For this review, take the finished solid that the model builds, in its own axes (mm). A direction names the side the tool comes from. Coordinates: 2 decimals unless noted, no trailing zeros. Write each loop counter-clockwise with the first axis right and the second up, starting at its lowest first coordinate (ties: lowest second). Pieces come first, ordered by that corner, then holes. Notation, with made-up numbers: (-22, 41.25) - (28, 41.25) arc R17 ccw to (28, 56.25) - close; hole circle Ø10 at (46, -25.5). An arc over 180 degrees is marked (long way). Write each question's results on one line, items separated by ' | '.
from build123d import *

# Parameters (mm, degrees)
SKETCH_1_W          = 41
SKETCH_1_H          = 19
EXTRUDE_2_DEPTH     = 2
SKETCH_2_W          = 41
SKETCH_2_H          = 2
EXTRUDE_3_DEPTH     = 25
SKETCH_3_R          = 2
CUT_EXTRUDE_1_DEPTH = 25
FILLET_1_R          = 1
FILLET_2_R          = 1
FILLET_3_R          = 1
FILLET_4_R          = 1
FILLET_5_R          = 1
FILLET_6_R          = 1


with BuildPart() as part:
    # 草图1 → 凸台-拉伸2 (new body)
    with BuildSketch(Plane(origin=(0, 0, 0), x_dir=(1, 0, 0), z_dir=(0, 1, 0))):
        Rectangle(SKETCH_1_W, SKETCH_1_H)
    extrude(amount=EXTRUDE_2_DEPTH)

    # 草图2 → 凸台-拉伸3 (add)
    with BuildSketch(Plane(origin=(0, 2, 0), x_dir=(1, 0, 0), z_dir=(0, 1, 0))):
        with Locations((0, 8.5)):
            Rectangle(SKETCH_2_W, SKETCH_2_H)
    extrude(amount=EXTRUDE_3_DEPTH)

    # 草图3 → 切除-拉伸1 (cut)
    with BuildSketch(Plane.XY.offset(-7.5)):
        with Locations((-12.5, 19)):
            Circle(SKETCH_3_R)
        with Locations((12.5, 19)):
            Circle(SKETCH_3_R)
    extrude(amount=-CUT_EXTRUDE_1_DEPTH, mode=Mode.SUBTRACT)

    # 圆角1
    fillet_1_edges = [part.edges().sort_by_distance(p)[0] for p in [
        (0, 2, -7.5),
    ]]
    fillet(fillet_1_edges, radius=FILLET_1_R)

    # 圆角2
    fillet_2_edges = [part.edges().sort_by_distance(p)[0] for p in [
        (0, 0, -9.5),
    ]]
    fillet(fillet_2_edges, radius=FILLET_2_R)

    # 圆角3
    fillet_3_edges = [part.edges().sort_by_distance(p)[0] for p in [
        (-20.5, 1, 9.5),
    ]]
    fillet(fillet_3_edges, radius=FILLET_3_R)

    # 圆角4
    fillet_4_edges = [part.edges().sort_by_distance(p)[0] for p in [
        (20.5, 1, 9.5),
    ]]
    fillet(fillet_4_edges, radius=FILLET_4_R)

    # 圆角5
    fillet_5_edges = [part.edges().sort_by_distance(p)[0] for p in [
        (-20.5, 27, -8.5),
    ]]
    fillet(fillet_5_edges, radius=FILLET_5_R)

    # 圆角6
    fillet_6_edges = [part.edges().sort_by_distance(p)[0] for p in [
        (20.5, 27, -8.5),
    ]]
    fillet(fillet_6_edges, radius=FILLET_6_R)


solid = part.part
Q1. Take a section at C-C on z = 7.5. State the section outline as (x, y) points.
Results found:
outline: (-20.5, 0) - (20.5, 0) - (20.5, 2) - (-20.5, 2) - close
Q2. Wall thickness on line 1 along Y through (x, z) = (-12.5, -8); line 2 along Z through (x, y) = (-6.5, 9.75); line 3 along Y through (x, z) = (4.5, -0.25): over which ranges is each line inside the solid? List them lowest first. Write a range as from..to.
Results found:
line 1: 0..17, 21..27 | line 2: -9.5..-7.5 | line 3: 0..2
Q3. Mouldability with a two-part tool opening along Y and no side actions: class faces 3 (the face through (0.287, 0.301, -9.215)), 4 (the face through (-20.5, 8, -8)), 5 (the face through (12.24, 20.983, -8.486)) as pulls with the +Y half, pulls with the -Y half, needs draft (parallel to the pull), parting line crosses it, or undercut.
Results found:
face 3: pulls with the -Y half | face 4: needs draft | face 5: undercut
Q4. Take a section at D-D on y = 14. State the section outline as (x, z) points.
Results found:
outline: (-20.5, -9.5) - (20.5, -9.5) - (20.5, -7.5) - (-20.5, -7.5) - close
Q5. For faces 1 (the face through (0, 2, 1)), 2 (the face through (0, 1, 9.5)), list the 3-axis set-ups (+Z, -Z, +X, -X, +Y, -Y) from which the entire face can be reached by the end or side of a thin tool; tool diameter is ignored.
Results found:
face 1: +Z, +X, -X, +Y | face 2: +Z, +X, -X, +Y, -Y
Q6. For pin 1 (8 mm diameter, centred on x = -9, z = 4.5, fed in from +Y); pin 2 (10 mm diameter, centred on y = 9, z = 4, fed in from +X), all flat-tipped, find the tip position at first contact; note any pin that passes through.
Results found:
pin 1: y = 2 | pin 2: through
Q7. Take a section at A-A on y = 19. State the section outline as (x, z) points, plus the area to 3 significant figures.
Results found:
outline: (-20.5, -9.5) - (-14.5, -9.5) - (-14.5, -7.5) - (-20.5, -7.5) - close; (-10.5, -9.5) - (10.5, -9.5) - (10.5, -7.5) - (-10.5, -7.5) - close; (14.5, -9.5) - (20.5, -9.5) - (20.5, -7.5) - (14.5, -7.5) - close | area: 66.0 mm2
Q8. Take a section at B-B on x = -12.5. State the section outline as (y, z) points, plus the area to 3 significant figures.
Results found:
outline: (0, -8.5) arc R1 ccw to (1, -9.5) - (17, -9.5) - (17, -7.5) - (3, -7.5) arc R1 cw to (2, -6.5) - (2, 9.5) - (0, 9.5) - close; (21, -9.5) - (27, -9.5) - (27, -7.5) - (21, -7.5) - close | area: 80.0 mm2
